Check sheet for the drawn part. Datum: minimum x, y, z corner. Units: mm. Round coordinates to 2 decimals unless told otherwise and drop trailing zeros. Write each loop counter-clockwise with the first axis right and the second up, starting at its lowest first coordinate (ties: lowest second). Pieces come first, ordered by that corner, then holes. Notation, with made-up numbers: (65, 28) - (100, 28) arc R19 ccw to (100, 64) - close; hole circle Ø4 at (11, 28). An arc over 180 degrees is marked (long way). Answer as a JSON object with one key per item and string values. Group by question number.
1) Go/stop test with flat-tipped pins: pin 1 Ø10 at (x, y) = (49, 148.5) entering from +Z; pin 2 Ø1 at (x, z) = (31, 106) entering from +Y. Record where each tip stops, or that it passes through.
2) Section check C-C (y = 145.5). Enter the section's corners in (x, z).
3) Thickness scan on line 1 (X direction, y = 217.5, z = 102); line 2 (Y direction, x = 156, z = 119.5); line 3 (Y direction, x = 70.5, z = 107.5). Record the ranges inside material, lowest first.
4) Section check B-B (z = 112.5). Enter the section's corners in (x, y).
5) Section check A-A (x = 157). Enter the section's corners in (y, z), then the cut area to 3 significant figures.
6) Section check D-D (x = 67). Enter the section's corners in (y, z).
7) Mould release check, pull along Y, two halves, no side actions. Record for the marked faces 1, 2, 3 and 4: +Y half, -Y half, draft (parallel to the pull), parting line (faces both ways), or undercut.
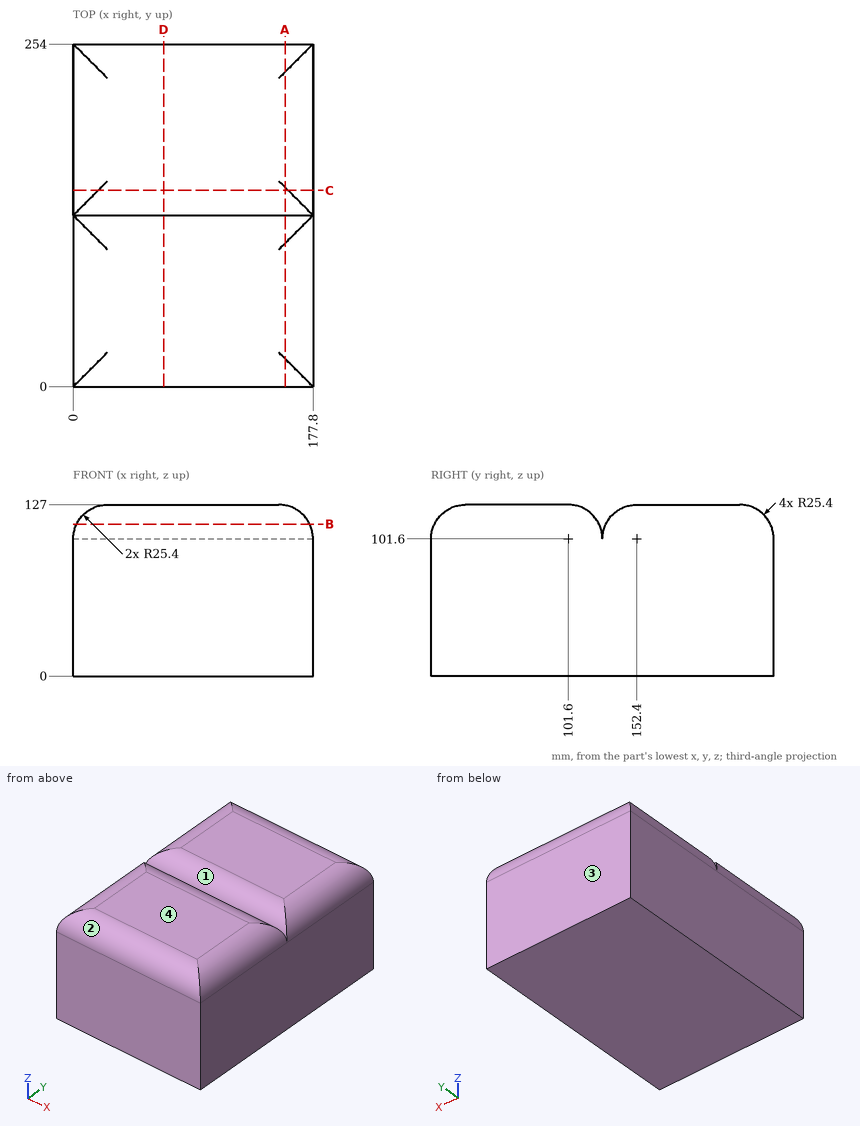
Returned:
{
 "1": {"pin 1": "z = 127", "pin 2": "y = 253.7"},
 "2": {"outline": "(0, 0) - (177.8, 0) - (177.8, 101.6) arc R25.4 ccw to (159.3, 126.04) - (18.5, 126.04) arc R25.4 ccw to (0, 101.6) - close"},
 "3": {"line 1": "0 to 177.8", "line 2": "7.38 to 119.62, 134.38 to 246.62", "line 3": "0.69 to 126.31, 127.69 to 253.31"},
 "4": {"outline": "(2.46, 2.46) - (175.34, 2.46) - (175.34, 124.54) - (2.46, 124.54) - close; (2.46, 129.46) - (175.34, 129.46) - (175.34, 251.54) - (2.46, 251.54) - close"},
 "5": {"outline": "(0, 0) - (254, 0) - (254, 101.6) arc R25.4 ccw to (233.2, 126.58) - (147.8, 126.58) arc R25.4 ccw to (127, 101.6) arc R25.4 ccw to (106.2, 126.58) - (20.8, 126.58) arc R25.4 ccw to (0, 101.6) - close", "area": "31,600 mm2"},
 "6": {"outline": "(0, 0) - (254, 0) - (254, 101.6) arc R25.4 ccw to (228.6, 127) - (152.4, 127) arc R25.4 ccw to (127, 101.6) arc R25.4 ccw to (101.6, 127) - (25.4, 127) arc R25.4 ccw to (0, 101.6) - close"},
 "7": {"face 1": "undercut", "face 2": "-Y half", "face 3": "+Y half", "face 4": "draft"}
}
